Verification items for the finished model (mm, model axes). A direction names the side the tool comes from. Coordinates: 2 decimals unless noted, no trailing zeros. Loops run counter-clockwise (first coordinate to the right, second up) from the corner with the lowest first, then second, coordinate; pieces in that order, holes last. Notation, with made-up numbers: (13, -30) -> (66, -30) arc R16 cw to (66, -10) -> close; hole circle Ø1 at (84, 78). An arc over 180 degrees is marked (long way). Use CSV: the item, a comma, the result in double quotes. Start each with the question number.
```python
from build123d import *

# Parameters (mm, degrees)
F1_DEPTH       = 20
F3_D           = 5
F3_CBORE_D     = 9.75
F3_CBORE_DEPTH = 9.5
F5_D           = 4.5
F5_DEPTH       = 10
F5_TIP         = 1.3519363928
F6_R           = 1.5
F7_DEPTH       = 25
F9_DEPTH       = 15.001
F10_SIZE       = 1


with BuildPart() as f1:
    # F0 (on Front) → F1 (new body)
    with BuildSketch(Plane.XZ):
        Polygon((7.5, 0), (-7.5, 0), (-7.5, -22), (7.5, -19.3550952894), align=None)
    extrude(amount=-F1_DEPTH)

    # F3 (through all)
    with Locations(Plane(origin=(-7.5, 0, 0), x_dir=(0, -1, 0), z_dir=(-1, 0, 0))):
        with Locations((-8, -8)):
            CounterBoreHole(F3_D / 2, F3_CBORE_D / 2, F3_CBORE_DEPTH)

    # F5
    with Locations(Plane(origin=(3.5360689045, 0, -20.0540432912), x_dir=(0.984807753, 0, 0.1736481777), z_dir=(0.1736481777, 0, -0.984807753))):
        with Locations((-3.5906184671, -16)):
            Hole(F5_D / 2, depth=F5_DEPTH)
            with Locations((0, 0, -(F5_DEPTH + F5_TIP / 2))):  # 118° drill point
                Cone(0, F5_D / 2, F5_TIP, mode=Mode.SUBTRACT)

    # F6 (on face) → F7 (cut)
    with BuildSketch(Plane(origin=(0, 20, 0), x_dir=(-1, 0, 0), z_dir=(0, 1, 0))):
        with Locations((3.5, -8)):
            Circle(F6_R)
    extrude(amount=-F7_DEPTH, mode=Mode.SUBTRACT)

    # F8 (on face) → F9 (cut, through all)
    with BuildSketch(Plane(origin=(-7.5, 0, 0), x_dir=(0, -1, 0), z_dir=(-1, 0, 0))):
        with BuildLine():
            Line((0, 0), (-8, 0))
            ThreePointArc((-8, 0), (-2.3431457505, -2.3431457505), (0, -8))
            Line((0, -8), (0, 0))
        make_face()
        with BuildLine():
            Line((-8, -17.3808315196), (-8, -22))
            Line((-8, -22), (0, -22))
            Line((0, -22), (0, -8))
            ThreePointArc((0, -8), (-1.912912718, -13.1910854762), (-6.7368421053, -15.8996475955))
            ThreePointArc((-6.7368421053, -15.8996475955), (-7.6413288654, -16.4075029929), (-8, -17.3808315196))
        make_face()
    extrude(amount=-F9_DEPTH, mode=Mode.SUBTRACT)

    # F10
    f10_edges = [f1.edges().sort_by_distance(p)[0] for p in [
        (7.5, 20, -9.677548),
        (-7.5, 20, -11),
        (-7.5, 14, 0),
        (-7.5, 8, -19.690416),
        (-7.5, 12.875, -8),
        (-7.5, 7.641329, -16.407503),
        (-7.5, 0.025128, -7.366431),
    ]]
    chamfer(f10_edges, length=F10_SIZE)


solid = f1.part
```
1. Scan lines: line 1 (X direction, y = 1.2, z = -8); line 2 (Y direction, x = -0.5, z = -8) (3 decimals); line 3 (Z direction, x = -4.25, y = 4.5). Record each from-to range of solid material in increasing order.
2. Release check for a two-part mould opening along Z. For faces 4 (the cylindrical face through (-2, 2, -8)), 5 (the conical face through (-2.01, 16.38, -9.74)), 6 (the flat face through (-7, 19.5, -10.8)), 7 (the flat face through (1, 14, 0)) record: released by +Z, released by -Z, zero draft, split by the parting line, or undercut.
3. Depth check by flat-ended pin: pin 1 (4.5 mm diameter, centred on y = 8, z = -8, fed in from -X); pin 2 (1.5 mm diameter, centred on y = 10.5, z = -12, fed in from -X); pin 3 (5 mm diameter, centred on x = 1, z = -19, fed in from -Y); pin 4 (4 mm diameter, centred on x = 4.5, z = -15.5, fed in from -Y). Enter the tip coordinate at first touch or a pass-through.
4. Set-up check for faces 1 (the flat face through (-7, 8.5, -19.7)), 2 (the flat face through (2, 6, -10)), 3 (the flat face through (-1, 8, -19)): record each of +Z, -Z, +X, -X, +Y, -Y from which the full face is reachable in a straight line by a thin tool's end or side.
5. Cross-section at B-B, the plane x = -3.5. State how many separate pieces and enclosed holes the cut face has, plus the area to 3 significant figures.
6. Cross-section at A-A, the plane z = -8. Record the boundary of the cut face in (x, y) (3 decimals).
Solution:
1,line 1,"x = -7.5 to -5, -2 to 7.5"
1,line 2,"y = 0 to 3.125, 12.875 to 20"
1,line 3,"z = -15.19 to -11.39, -4.61 to -0.81"
2,face 4,"undercut"
2,face 5,"undercut"
2,face 6,"zero draft"
2,face 7,"released by +Z"
3,pin 1,"passes through"
3,pin 2,"stops at x = -7.09"
3,pin 3,"stops at y = 7.71"
3,pin 4,"stops at y = 2.19"
4,face 1,"-Z, -X, -Y"
4,face 2,"-X"
4,face 3,"-Z, +X, -X, -Y"
5,separate pieces,"2"
5,enclosed holes,"1"
5,area,"245 mm2"
6,outline,"(-7.5, 1) -> (-6.5, 0) -> (-5, 0) -> (-5, 3.125) -> (-6.5, 3.125) -> (-7.5, 2.125) -> close; (-7.5, 13.875) -> (-6.5, 12.875) -> (-5, 12.875) -> (-5, 20) -> (-6.5, 20) -> (-7.5, 19) -> close; (-2, 0) -> (7.5, 0) -> (7.5, 5.5) -> (2, 5.5) -> (2, 3.125) -> (-2, 3.125) -> close; (-2, 12.875) -> (2, 12.875) -> (2, 10.5) -> (7.5, 10.5) -> (7.5, 19) -> (6.5, 20) -> (-2, 20) -> close"
